Could you check a few things on this model? Use its own coordinates, in mm. A direction names the side the tool comes from. Round coordinates to 2 decimals unless told otherwise and drop trailing zeros. Write each loop counter-clockwise with the first axis right and the second up, starting at its lowest first coordinate (ties: lowest second). Pieces come first, ordered by that corner, then holes. Notation, with made-up numbers: (77.5, -28) - (98.5, -28) arc R31 ccw to (98.5, -3) - close; hole circle Ø5 at (19.25, 0). An arc over 180 degrees is marked (long way). Put each result on its own line as item: value.
from build123d import *

# Parameters (mm, degrees)
SKETCH1_W               = 110
SKETCH1_H               = 45
SKETCH1_R               = 15
SKETCH1_R_2             = 3
BOSS_EXTRUDE1_DEPTH     = 45
CUT_EXTRUDE4_REACH      = 129.083
CUT_EXTRUDE4_END_RADIUS = 15
BOSS_EXTRUDE2_DEPTH     = 4.5
BOSS_EXTRUDE3_DEPTH     = 4.5
SKETCH12_R              = 3
CUT_EXTRUDE5_DEPTH      = 4.5
SKETCH15_R              = 3
CUT_EXTRUDE6_DEPTH      = 4.5
SKETCH16_R              = 6
CUT_EXTRUDE7_DEPTH      = 1
SKETCH18_W              = 38
SKETCH18_H              = 12
CUT_EXTRUDE8_DEPTH      = 128.082650271


with BuildPart() as part:
    # Sketch1 → Boss-Extrude1 (new body)
    with BuildSketch(Plane.XY):
        with Locations((55, 22.5)):
            Rectangle(SKETCH1_W, SKETCH1_H)
        with Locations(Location((50, 20, 0), (0, 0, 180))):
            Circle(SKETCH1_R, mode=Mode.SUBTRACT)
        with Locations(Location((80, 28, 0), (0, 0, 180))):
            Circle(SKETCH1_R_2, mode=Mode.SUBTRACT)
        with BuildLine():
            ThreePointArc((80, 5), (96.263455967, 11.736544033), (103, 28))
            ThreePointArc((103, 28), (100, 31), (97, 28))
            ThreePointArc((97, 28), (92.02081528, 15.97918472), (80, 11))
            ThreePointArc((80, 11), (77, 8), (80, 5))
        make_face(mode=Mode.SUBTRACT)
    boss_extrude1 = extrude(amount=BOSS_EXTRUDE1_DEPTH)

    # Cut-Extrude4: up to this cylinder (the profile starts outside it)
    cut_extrude4_end = Plane(origin=(50, 20, 22.5), z_dir=(0, 0, -1)) * Cylinder(CUT_EXTRUDE4_END_RADIUS, 308.166, mode=Mode.PRIVATE)
    # Sketch3 → Cut-Extrude4 (cut, up to the surface)
    with BuildSketch(Plane(origin=(0, 45, 0), x_dir=(1, 0, 0), z_dir=(0, 1, 0)), mode=Mode.PRIVATE) as cut_extrude4_sk1:
        Polygon((55.485397506, -32), (52.59864616, -27), (46.825143468, -27), (43.938392122, -32), (46.825143468, -37), (52.59864616, -37), align=None)
    cut_extrude4_tool1 = extrude(cut_extrude4_sk1.sketch, amount=-CUT_EXTRUDE4_REACH, mode=Mode.PRIVATE) - cut_extrude4_end
    add(cut_extrude4_tool1.solids().sort_by_distance((49.711895, 45, 32))[0], mode=Mode.SUBTRACT)
    # Sketch3 → Cut-Extrude4 (cut, up to the surface)
    with BuildSketch(Plane(origin=(0, 45, 0), x_dir=(1, 0, 0), z_dir=(0, 1, 0)), mode=Mode.PRIVATE) as cut_extrude4_sk2:
        Polygon((55.485397506, -13), (52.59864616, -8), (46.825143468, -8), (43.938392122, -13), (46.825143468, -18), (52.59864616, -18), align=None)
    cut_extrude4_tool2 = extrude(cut_extrude4_sk2.sketch, amount=-CUT_EXTRUDE4_REACH, mode=Mode.PRIVATE) - cut_extrude4_end
    add(cut_extrude4_tool2.solids().sort_by_distance((49.711895, 45, 13))[0], mode=Mode.SUBTRACT)

    # Sketch9 → Boss-Extrude2 (add)
    with BuildSketch(Plane(origin=(0, 45, 0), x_dir=(1, 0, 0), z_dir=(0, 1, 0))):
        Polygon((46.825143468, -8), (43.938392122, -13), (46.825143468, -18), (52.59864616, -18), (55.485397506, -13), (52.59864616, -8), align=None)
    extrude(amount=-BOSS_EXTRUDE2_DEPTH)

    # Sketch10 → Boss-Extrude3 (add)
    with BuildSketch(Plane(origin=(0, 45, 0), x_dir=(1, 0, 0), z_dir=(0, 1, 0))):
        Polygon((43.938392122, -32), (46.825143468, -37), (52.59864616, -37), (55.485397506, -32), (52.59864616, -27), (46.825143468, -27), align=None)
    extrude(amount=-BOSS_EXTRUDE3_DEPTH)

    # Sketch12 → Cut-Extrude5 (cut)
    with BuildSketch(Plane.XZ.offset(-40.5)):
        with Locations(Location((49.576462362, 13, 0), (0, 0, 270))):
            Circle(SKETCH12_R)
    cut_extrude5 = extrude(amount=-CUT_EXTRUDE5_DEPTH, mode=Mode.SUBTRACT)

    # Sketch15 → Cut-Extrude6 (cut)
    with BuildSketch(Plane.XZ.offset(-40.5)):
        with Locations(Location((49.63041025, 32, 0), (0, 0, 270))):
            Circle(SKETCH15_R)
    cut_extrude6 = extrude(amount=-CUT_EXTRUDE6_DEPTH, mode=Mode.SUBTRACT)

    # Sketch16 → Cut-Extrude7 (cut)
    with BuildSketch(Plane(origin=(0, 45, 0), x_dir=(1, 0, 0), z_dir=(0, 1, 0))):
        with Locations(Location((49.63041025, -32, 0), (0, 0, 270))):
            Circle(SKETCH16_R)
        with Locations(Location((49.576462362, -13, 0), (0, 0, 270))):
            Circle(SKETCH16_R)
    cut_extrude7 = extrude(amount=-CUT_EXTRUDE7_DEPTH, mode=Mode.SUBTRACT)

    # Sketch18 → Cut-Extrude8 (cut, through all)
    with BuildSketch(Plane(origin=(0, 45, 0), x_dir=(1, 0, 0), z_dir=(0, 1, 0))):
        with Locations((91, -22.5)):
            Rectangle(SKETCH18_W, SKETCH18_H)
    cut_extrude8 = extrude(amount=-CUT_EXTRUDE8_DEPTH, mode=Mode.SUBTRACT)

    # Mirror1: Boss-Extrude1, Cut-Extrude5, Cut-Extrude6, Cut-Extrude7, Cut-Extrude8 across plane
    add(boss_extrude1.mirror(Plane(origin=(0, 0, 45), x_dir=(0, 0, 1), z_dir=(-1, 0, 0))))
    add(cut_extrude5.mirror(Plane(origin=(0, 0, 45), x_dir=(0, 0, 1), z_dir=(-1, 0, 0))), mode=Mode.SUBTRACT)
    add(cut_extrude6.mirror(Plane(origin=(0, 0, 45), x_dir=(0, 0, 1), z_dir=(-1, 0, 0))), mode=Mode.SUBTRACT)
    add(cut_extrude7.mirror(Plane(origin=(0, 0, 45), x_dir=(0, 0, 1), z_dir=(-1, 0, 0))), mode=Mode.SUBTRACT)
    add(cut_extrude8.mirror(Plane(origin=(0, 0, 45), x_dir=(0, 0, 1), z_dir=(-1, 0, 0))), mode=Mode.SUBTRACT)


solid = part.part
(1) Imagine slicing it at B-B, the plane x = -63. List the corners of the cut face in (y, z) for me.
Values found:
outline: (0, 0) - (12.52, 0) - (12.52, 45) - (0, 45) - close; (27.48, 0) - (45, 0) - (45, 45) - (27.48, 45) - close
(2) Imagine slicing it at D-D, the plane y = 8. Give the number of separate pieces and of enclosed holes in the cut face, then the cut area to 3 significant figures.
Values found:
separate pieces: 7
enclosed holes: 0
area: 6,420 mm^2
(3) For faces 1 (the face through (72, 23, 23)), 2 (the face through (52.2, 40.5, 34.2)), 3 (the face through (-91, 23, 28.5)), 4 (the face through (96.084, 11.559, 36.634)), which set-ups out of +Z, -Z, +X, -X, +Y, -Y let a thin tool reach every point of the face, with its end or its side?
Values found:
face 1: +X, +Y, -Y
face 2: none
face 3: -X, +Y, -Y
face 4: +Z, -Z
(4) I'm going to push flat-ended pins straight in: pin 1 (9.5 mm diameter, centred on x = -80, y = 28, fed in from +Z); pin 2 (6 mm diameter, centred on x = -47.5, z = 11.5, fed in from +Y); pin 3 (4 mm diameter, centred on y = 26, z = 24.5, fed in from +X). Where does each tip first touch, or does it pass through?
Values found:
pin 1: stops at z = 45
pin 2: stops at y = 44
pin 3: stops at x = 72
(5) Imagine slicing it at A-A, the plane z = 5. List the corners of the cut face in (x, y) for me.
Values found:
outline: (-110, 0) - (110, 0) - (110, 45) - (-110, 45) - close; hole (-103, 28) arc R23 ccw to (-80, 5) arc R3 ccw to (-80, 11) arc R17 cw to (-97, 28) arc R3 ccw to start; hole circle Ø6 at (-80, 28); hole circle Ø30 at (-50, 20); hole circle Ø30 at (50, 20); hole circle Ø6 at (80, 28); hole (80, 5) arc R23 ccw to (103, 28) arc R3 ccw to (97, 28) arc R17 cw to (80, 11) arc R3 ccw to start
(6) If we mould it in two halves opening along Y, with no side actions, what happens to faces 5 (the face through (51.604, 42.226, 15.211)), 6 (the face through (-77, 8, 8)), 7 (the face through (-100, 31, 8)), 8 (the face through (-50, 40.5, 32))? For each: pulls with the +Y half, pulls with the -Y half, needs draft (parallel to the pull), parting line crosses it, or undercut.
Values found:
face 5: needs draft
face 6: undercut
face 7: undercut
face 8: pulls with the +Y half
(7) Please list where these lines run through material, in increasing order: probe 1 along Y at (x, z) = (80, 6); probe 2 along X at (y, z) = (41, 13); probe 3 along Z at (x, y) = (-91.5, 29). Write a range as from..to.
Values found:
probe 1: y = 0..5, 11..25, 31..45
probe 2: x = -110..-52.58, -46.58..46.58, 52.58..110
probe 3: z = 0..16.5, 28.5..45
(8) Imagine slicing it at C-C, the plane x = 92. List the corners of the cut face in (y, z) for me.
Values found:
outline: (0, 0) - (8.38, 0) - (8.38, 16.5) - (0, 16.5) - close; (0, 28.5) - (8.38, 28.5) - (8.38, 45) - (0, 45) - close; (15.96, 0) - (45, 0) - (45, 16.5) - (15.96, 16.5) - close; (15.96, 28.5) - (45, 28.5) - (45, 45) - (15.96, 45) - close
